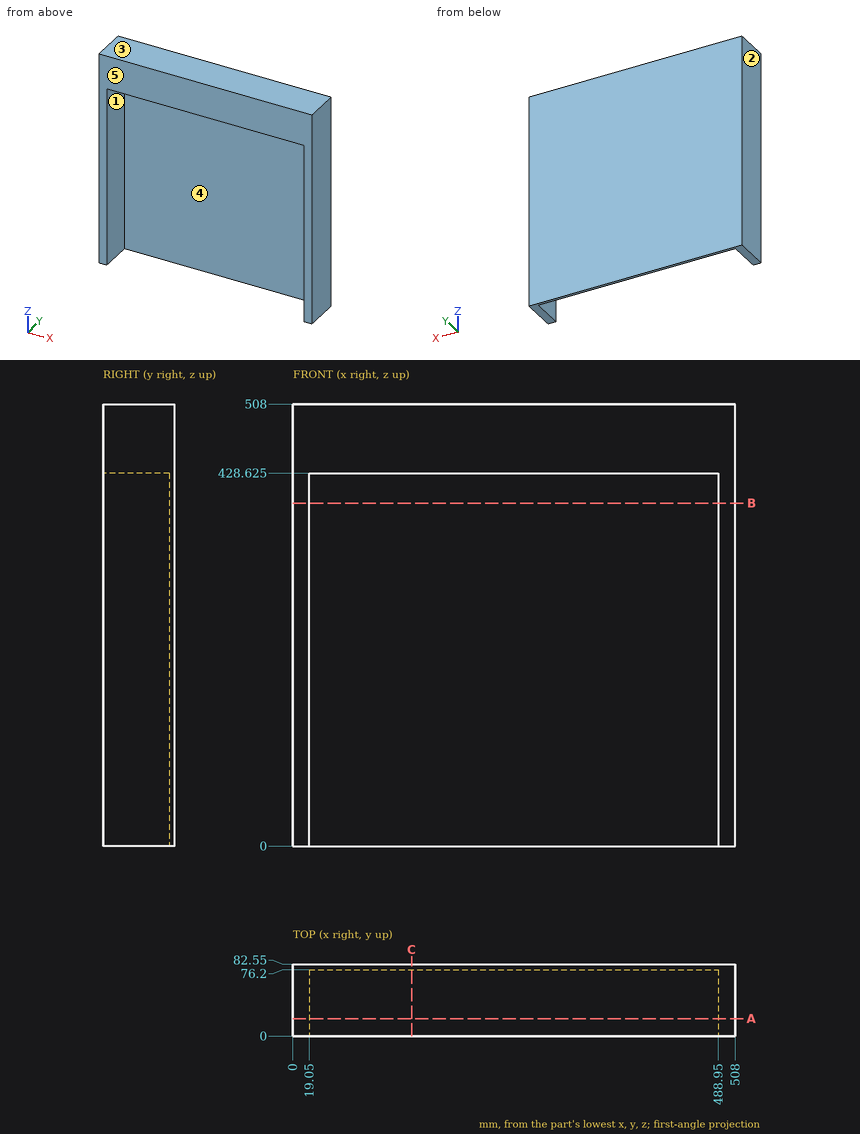
Job drawing, mm, ordinate dimensions from the low corner. One solid piece. A direction names the side the tool comes from. Round coordinates to 2 decimals unless told otherwise and drop trailing zeros. Loops run counter-clockwise (first coordinate to the right, second up) from the corner with the lowest first, then second, coordinate; pieces in that order, holes last. Notation, with made-up numbers: (-35, 16.5) -> (-14, 16.5) arc R17 cw to (-14, 46.5) -> close; hole circle Ø1 at (0, 22). An arc over 180 degrees is marked (long way). One line per item, written item: value. Start each with the question number.
Q1. Cut at A-A on y = 20. List the corners of the cut face in (x, z) (3 decimals).
Q2. 3-axis set-ups, long thin cutter, end or side, ignore diameter. For the marked faces 4 and 5: which of +Z, -Z, +X, -X, +Y, -Y reach the whole face in a straight line?
Q3. Two-plate mould, pull along X, no slides. Class the marked faces 1, 2 and 3: released by +X, released by -X, zero draft, split by the parting line, or undercut.
Q4. Cut at B-B on z = 394. List the corners of the cut face in (x, y), plus the area to 3 significant figures.
Q5. Cut at C-C on x = 136.5. List the corners of the cut face in (y, z) (3 decimals), plus the area to 3 significant figures.
Q6. Drop flat-ended pins along their axis: pin 1 Ø12 at (x, y) = (76, 65) entering from -Z (3 decimals); pin 2 Ø10 at (x, z) = (312.5, 71.5) entering from -Y. Give the stop position or say it passes through.
Q7. Probe line 1 along X through (y, z) = (37.5, 99.5); line 2 along Z through (x, y) = (417.5, 28.5) (3 decimals); line 3 along Y through (x, z) = (181, 190). List the from-to ranges inside material, lowest first.
Computed:
1. outline: (0, 0) -> (19.05, 0) -> (19.05, 428.625) -> (488.95, 428.625) -> (488.95, 0) -> (508, 0) -> (508, 508) -> (0, 508) -> close
2. face 4: -Z, -Y
2. face 5: +Z, -Z, +X, -X, -Y
3. face 1: undercut
3. face 2: released by -X
3. face 3: zero draft
4. outline: (0, 0) -> (19.05, 0) -> (19.05, 76.2) -> (488.95, 76.2) -> (488.95, 0) -> (508, 0) -> (508, 82.55) -> (0, 82.55) -> close
4. area: 6,130 mm²
5. outline: (0, 428.625) -> (76.2, 428.625) -> (76.2, 0) -> (82.55, 0) -> (82.55, 508) -> (0, 508) -> close
5. area: 9,270 mm²
6. pin 1: z = 428.625
6. pin 2: y = 76.2
7. line 1: 0 to 19.05, 488.95 to 508
7. line 2: 428.625 to 508
7. line 3: 76.2 to 82.55
